from build123d import *

# Parameters (mm, degrees)
SKETCH1_W           = 100
SKETCH1_H           = 100
BOSS_EXTRUDE1_DEPTH = 10
SKETCH2_R           = 2
CUT_EXTRUDE1_DEPTH  = 72.414284285
SKETCH3_R           = 7.65
SKETCH3_R_2         = 5.15
EXTRUDE_THIN1_DEPTH = 20
RIB1_START          = -1.5
RIB1_DEPTH          = 3
CIRPATTERN1_COUNT   = 4
FILLET1_R           = 5
CUT_EXTRUDE3_DEPTH  = 7


with BuildPart() as part:
    # Sketch1 → Boss-Extrude1 (new body)
    with BuildSketch(Plane(origin=(0, 0, 0), x_dir=(1, 0, 0), z_dir=(0, 1, 0))):
        Rectangle(SKETCH1_W, SKETCH1_H)
    extrude(amount=BOSS_EXTRUDE1_DEPTH)

    # Sketch2 → Cut-Extrude1 (cut, through all)
    with BuildSketch(Plane(origin=(0, 10, 0), x_dir=(1, 0, 0), z_dir=(0, 1, 0))):
        with Locations(Location((-45, 35, 0), (0, 0, 270))):
            Circle(SKETCH2_R)
        with Locations(Location((45, 35, 0), (0, 0, 270))):
            Circle(SKETCH2_R)
        with Locations(Location((45, -35, 0), (0, 0, 270))):
            Circle(SKETCH2_R)
        with Locations(Location((-45, -35, 0), (0, 0, 270))):
            Circle(SKETCH2_R)
    extrude(amount=-CUT_EXTRUDE1_DEPTH, mode=Mode.SUBTRACT)

    # Sketch3 → Extrude-Thin1 (add)
    with BuildSketch(Plane(origin=(0, 10, 0), x_dir=(1, 0, 0), z_dir=(0, 1, 0))):
        Circle(SKETCH3_R)
        Circle(SKETCH3_R_2, mode=Mode.SUBTRACT)
    extrude(amount=EXTRUDE_THIN1_DEPTH)

    # Rib1: read off the stored shape, not the designer's step
    # Rib1 outline → Rib1 (add)
    with BuildSketch(Plane.XY.offset(RIB1_START)):
        Polygon((-7.50149985, 30), (-7.65, 30), (-22.65, 10), (-7.50149985, 10), align=None)
    rib1 = extrude(amount=RIB1_DEPTH)

    # CirPattern1: Rib1 ×4 about axis
    cirpattern1_axis = Axis((0, 0, 0), (0, 1, 0))
    for i in range(1, CIRPATTERN1_COUNT):
        add(rib1.rotate(cirpattern1_axis, i * 360 / CIRPATTERN1_COUNT))

    # Fillet1
    fillet1_edges = [part.edges().sort_by_distance(p)[0] for p in [
        (50, 5, 50),
        (-50, 5, 50),
        (-50, 5, -50),
        (50, 5, -50),
    ]]
    fillet(fillet1_edges, radius=FILLET1_R)

    # Sketch6 → Cut-Extrude3 (cut)
    with BuildSketch(Plane.XZ):
        Polygon((4.67653718, -8.1), (9.353074361, 0), (4.67653718, 8.1), (-4.67653718, 8.1), (-9.353074361, 0), (-4.67653718, -8.1), align=None)
    extrude(amount=-CUT_EXTRUDE3_DEPTH, mode=Mode.SUBTRACT)


solid = part.part
The model under review builds one solid part; all positions refer to its coordinate system, in mm. A direction names the side the tool comes from. Give positions to 0.01 mm unless a question says otherwise; leave off trailing zeros. Write each loop counter-clockwise with the first axis right and the second up, starting at its lowest first coordinate (ties: lowest second). Pieces come first, ordered by that corner, then holes.
1. Add section A-A, the plane y = 19. Write out the cut boundary in (x, z), plus the area to 3 significant figures.
2. Wall thickness on L1, parallel to X at y = 3.75, z = -35; L2, parallel to Y at x = 4, z = 15.5; L3, parallel to Z at x = 16, y = 11: over which ranges is each line inside the solid? List them lowest first.
3. Tool access review of faces 4 (the cylindrical face through (5.454, 19.86, -5.365)), 5 (the cylindrical face through (5.365, 19.86, 5.454)), 6 (the cylindrical face through (4.91, 19.86, -1.55)): name each direction out of +Z, -Z, +X, -X, +Y, -Y from which nothing blocks a thin tool from reaching the whole face with its end or side.
4. Add section D-D, the plane x = 0. Write out the cut boundary in (y, z), plus the area to 3 significant figures.
5. Add section C-C, the plane y = 5.75. Write out the cut boundary in (x, z), plus the area to 3 significant figures.
6. For P1, Ø7.5, axis at x = 12.5, y = 20, coming from the -Z side; P2, Ø5, axis at x = 45, z = 35, coming from the +Y side; P3, Ø16.5, axis at x = 13.5, y = 22, coming from the +Z side; P4, Ø3, axis at x = -45, z = -35, coming from the +Y side, all flat-tipped, find the tip position at first contact; note any pin that passes through.
7. Add section B-B, the plane z = -35. Write out the cut boundary in (x, y).
8. Draft analysis for pull direction Z (two halves, no side actions). For faces 1 (the cylindrical face through (49, 5, 48)), 2 (the flat face through (1.5, 16, 12)), 3 (the flat face through (-6.98, 3.45, 4.11)), state which applies: +Z half, -Z half, draft (parallel to the pull), parting line (faces both ways), or undercut.
Worked answers:
1. outline: (-15.9, -1.5) - (-7.5, -1.5) arc R7.65 ccw to (-1.5, -7.5) - (-1.5, -15.9) - (1.5, -15.9) - (1.5, -7.5) arc R7.65 ccw to (7.5, -1.5) - (15.9, -1.5) - (15.9, 1.5) - (7.5, 1.5) arc R7.65 ccw to (1.5, 7.5) - (1.5, 15.9) - (-1.5, 15.9) - (-1.5, 7.5) arc R7.65 ccw to (-7.5, 1.5) - (-15.9, 1.5) - close; hole circle Ø10.3 at (0, 0)
1. area: 200 mm2
2. L1: x = -50 to -47, -43 to 43, 47 to 50
2. L2: y = 0 to 10
2. L3: z = -1.5 to 1.5
3. face 4: -Z, +X, +Y
3. face 5: +Z, +X, +Y
3. face 6: +Y
4. outline: (0, -50) - (10, -50) - (10, -22.65) - (30, -7.65) - (30, -5.15) - (10, -5.15) - (10, 5.15) - (30, 5.15) - (30, 7.65) - (10, 22.65) - (10, 50) - (0, 50) - (0, 8.1) - (7, 8.1) - (7, -8.1) - (0, -8.1) - close
4. area: 1,290 mm2
5. outline: (-50, -45) arc R5 ccw to (-45, -50) - (45, -50) arc R5 ccw to (50, -45) - (50, 45) arc R5 ccw to (45, 50) - (-45, 50) arc R5 ccw to (-50, 45) - close; hole circle Ø4 at (-45, -35); hole circle Ø4 at (-45, 35); hole (-9.35, 0) - (-4.68, -8.1) - (4.68, -8.1) - (9.35, 0) - (4.68, 8.1) - (-4.68, 8.1) - close; hole circle Ø4 at (45, -35); hole circle Ø4 at (45, 35)
5. area: 9,700 mm2
6. P1: stops at z = -1.5
6. P2: stops at y = 10
6. P3: stops at z = 5.56
6. P4: passes through
7. outline: (-50, 0) - (-47, 0) - (-47, 10) - (-50, 10) - close; (-43, 0) - (43, 0) - (43, 10) - (-43, 10) - close; (47, 0) - (50, 0) - (50, 10) - (47, 10) - close
8. face 1: +Z half
8. face 2: draft
8. face 3: undercut
